Input: part model. Units: mm. Frame: model coordinates. A direction names the side the tool comes from. Coordinates: 2 decimals unless noted, no trailing zeros. Order: outer loops, then holes, each group sorted by start corner. A loop starts at its lowest first (then second) coordinate and runs counter-clockwise, first axis right, second up. Notation, with made-up numbers: (39.25, 77.25) - (59.25, 77.25) arc R27 cw to (59.25, 95.25) - close; hole circle Ø10 at (-9.75, 35.25). An arc over 180 degrees is marked (long way). Use a Markdown table: item, result. Add a question column.
from build123d import *

# Parameters (mm, degrees)
PAD_DEPTH       = 76.2
SKETCH001_W     = 10.962794
SKETCH001_H     = 10.668
POCKET_DEPTH    = 12.7
SKETCH002_R     = 1.27
POCKET001_DEPTH = 21.945587
FILLET_R        = 2.54
FILLET001_R     = 1.27


with BuildPart() as part:
    # Sketch → Pad (new body)
    with BuildSketch(Plane.YZ):
        with BuildLine():
            Line((0, 0), (-1.651, 0))
            ThreePointArc((-20.274588, 0), (-10.962794, -10.668), (-1.651, 0))
            Line((-21.944587, 0), (-20.274588, 0))
            Line((-21.944587, -17.018), (-21.944587, 0))
            Line((0, -17.018), (-21.944587, -17.018))
            Line((0, 0), (0, -17.018))
        make_face()
    extrude(amount=PAD_DEPTH)

    # Sketch001 → Pocket (cut, symmetric)
    with BuildSketch(Plane.YZ.offset(38.1)):
        with Locations((-5.481397, -5.334)):
            Rectangle(SKETCH001_W, SKETCH001_H)
    extrude(amount=POCKET_DEPTH, both=True, mode=Mode.SUBTRACT)

    # Sketch002 → Pocket001 (cut, through all)
    with BuildSketch(Plane.XZ):
        with Locations((38.1, -13.843)):
            Circle(SKETCH002_R)
    extrude(amount=POCKET001_DEPTH, mode=Mode.SUBTRACT)

    # Fillet
    fillet_edges = [part.edges().sort_by_distance(p)[0] for p in [
        (0, -21.109587, 0),
        (0, -0.8255, 0),
        (76.2, -0.8255, 0),
        (76.2, -21.109587, 0),
        (25.4, -0.8255, 0),
        (50.8, -0.8255, 0),
        (0, -10.972294, -17.018),
        (76.2, -10.972294, -17.018),
    ]]
    fillet(fillet_edges, radius=FILLET_R)

    # Fillet001
    fillet001_edges = [part.edges().sort_by_distance(p)[0] for p in [
        (0, -21.944587, -8.509),
    ]]
    fillet(fillet001_edges, radius=FILLET001_R)


solid = part.part
1) Cut plane C-C (y = -15). Return the cut outline in (x, z), and give its area (3 significant figures).
2) Reachability of faces 1 (the cylindrical face through (0.724, -20.516, -0.764)), 2 (the flat face through (38, -6, -10.668)) from +Z, -Z, +X, -X, +Y, -Y: full face, straight path, thin tool, end or side. Return the list, or none.
3) Pull-direction query (X, two-part tool) for faces 3 (the flat face through (63, -1, 0)), 4 (the cylindrical face through (0.764, -0.837, -0.724)), 5 (the flat face through (25.4, -3, -8)); classes: pulls with the +X half, pulls with the -X half, needs draft (parallel to the pull), parting line crosses it, or undercut.
4) Cut plane B-B (z = -3.25). Return the cut outline in (x, y), and give its area (3 significant figures).
5) Cut plane A-A (x = 38.1). Return the cut outline in (y, z), and give its area (3 significant figures).
6) Cut plane D-D (x = 13). Return the cut outline in (y, z), and give its area (3 significant figures).
7) Material intervals for L1, parallel to Z at x = 38.1, y = -4.5; L2, parallel to X at y = -0.75, z = -9.5; L3, parallel to Z at x = 44, y = -9.5, sorted ascending.
8) Contact query for flat-ended pins moving along their axis: P1, Ø2, axis at x = 13, y = -5.5, coming from the +Z side; P2, Ø3.5, axis at x = 38.1, z = -13.843, coming from the +Y side; P3, Ø3.5, axis at x = 34, y = -4.5, coming from the +Z side; P4, Ø8, axis at x = 30, y = -8, coming from the +Z side. Output: stop coordinate, or through.
Computed:
| question | item | result |
|---|---|---|
| 1 | outline | (0, -14.48) arc R2.54 ccw to (2.54, -17.02) - (73.66, -17.02) arc R2.54 ccw to (76.2, -14.48) - (76.2, -9.76) - (0, -9.76) - close; hole circle Ø2.54 at (38.1, -13.84) |
| 1 | area | 545 mm2 |
| 2 | face 1 | +Z, -X, +Y, -Y |
| 2 | face 2 | +Z, +Y |
| 3 | face 3 | needs draft |
| 3 | face 4 | pulls with the -X half |
| 3 | face 5 | undercut |
| 4 | outline | (0, -20.67) arc R1.27 ccw to (1.27, -21.94) - (74.93, -21.94) arc R1.27 ccw to (76.2, -20.67) - (76.2, -20.15) - (0, -20.15) - close; (0, -1.78) - (25.4, -1.78) - (25.4, 0) - (0, 0) - close; (50.8, -1.78) - (76.2, -1.78) - (76.2, 0) - (50.8, 0) - close |
| 4 | area | 226 mm2 |
| 5 | outline | (-21.94, -15.75) arc R1.27 ccw to (-20.67, -17.02) - (0, -17.02) - (0, -15.11) - (-21.94, -15.11) - close; (-21.94, -12.57) - (0, -12.57) - (0, -10.67) - (-10.96, -10.67) arc R9.4 cw to (-20.27, 0) - (-20.67, 0) arc R1.27 ccw to (-21.94, -1.27) - close |
| 5 | area | 119 mm2 |
| 6 | outline | (-21.94, -15.75) arc R1.27 ccw to (-20.67, -17.02) - (0, -17.02) - (0, 0) - (-1.65, 0) arc R9.4 cw (long way) to (-20.27, 0) - (-20.67, 0) arc R1.27 ccw to (-21.94, -1.27) - close |
| 6 | area | 210 mm2 |
| 7 | L1 | z = -17.02 to -15.11, -12.57 to -10.67 |
| 7 | L2 | x = 0 to 25.4, 50.8 to 76.2 |
| 7 | L3 | z = -17.02 to -10.67 |
| 8 | P1 | stops at z = -8.09 |
| 8 | P2 | stops at y = 0 |
| 8 | P3 | stops at z = -10.67 |
| 8 | P4 | stops at z = -10.61 |
